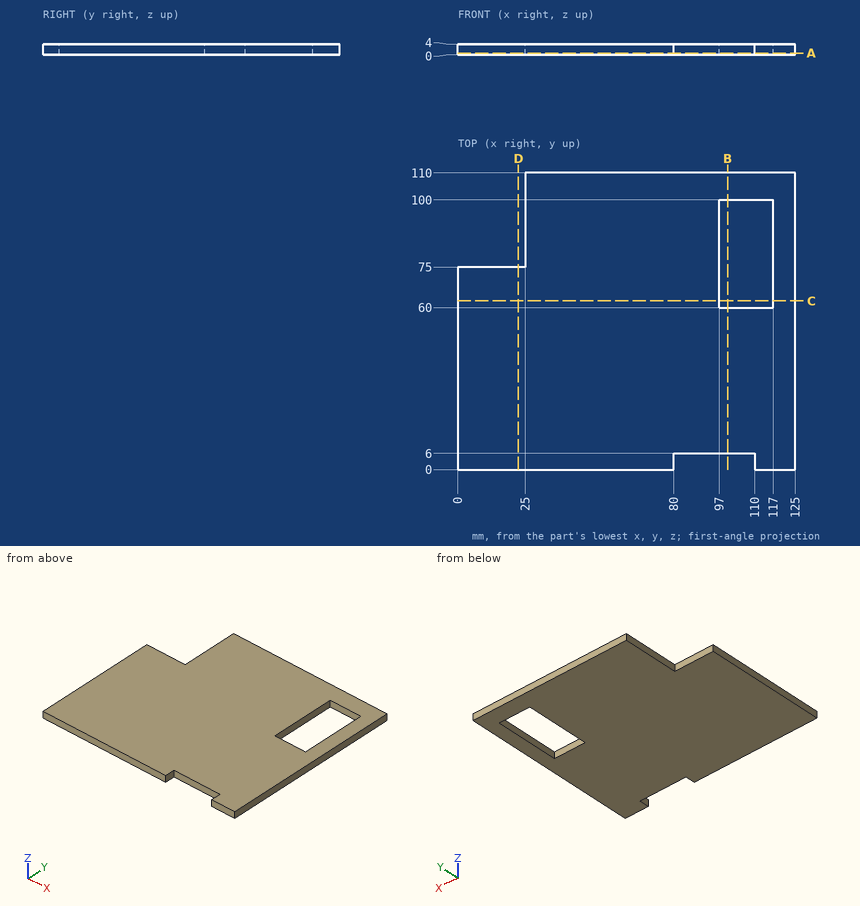
The figure shows three views and two pictorial views of one solid part (mm, origin at its lowest corner). Answer the questions. Coordinates: 2 decimals unless noted, no trailing zeros. Write each loop counter-clockwise with the first axis right and the second up, starting at its lowest first coordinate (ties: lowest second). Pieces come first, ordered by that corner, then holes.
1. The part is cut by section A-A, the plane z = 0.6. Write down the section's boundary in (x, y), and give its area (3 significant figures).
Results list:
outline: (0, 0) - (80, 0) - (80, 6) - (110, 6) - (110, 0) - (125, 0) - (125, 110) - (25, 110) - (25, 75) - (0, 75) - close; hole (97, 60) - (117, 60) - (117, 100) - (97, 100) - close
area: 11,900 mm2
2. The part is cut by section D-D, the plane x = 22.5. Write down the section's boundary in (y, z), and give its area (3 significant figures).
Results list:
outline: (0, 0) - (75, 0) - (75, 4) - (0, 4) - close
area: 300 mm2
3. The part is cut by section C-C, the plane y = 62.5. Write down the section's boundary in (x, z), and give its area (3 significant figures).
Results list:
outline: (0, 0) - (97, 0) - (97, 4) - (0, 4) - close; (117, 0) - (125, 0) - (125, 4) - (117, 4) - close
area: 420 mm2
4. Consider line 1 along X through (y, z) = (85.5, 0.45); line 2 along X through (y, z) = (70.5, 1.3); line 3 along Y through (x, z) = (23, 1.8). Determine where each line is inside the solid, lowest interval first.
Results list:
line 1: x = 25 to 97, 117 to 125
line 2: x = 0 to 97, 117 to 125
line 3: y = 0 to 75
5. Flat-ended cylindrical pins translate along their axes: pin 1 (1 mm diameter, centred on x = 12.5, z = 1, fed in from -Y); pin 2 (1.2 mm diameter, centred on y = 86.5, z = 2, fed in from -X); pin 3 (2 mm diameter, centred on x = 104, z = 1, fed in from -Y); pin 4 (2 mm diameter, centred on x = 17.5, z = 2, fed in from +Y). Find the tip coordinate at first contact, or state that the pin passes through.
Results list:
pin 1: stops at y = 0
pin 2: stops at x = 25
pin 3: stops at y = 6
pin 4: stops at y = 75
6. The part is cut by section B-B, the plane x = 100. Write down the section's boundary in (y, z), and give its area (3 significant figures).
Results list:
outline: (6, 0) - (60, 0) - (60, 4) - (6, 4) - close; (100, 0) - (110, 0) - (110, 4) - (100, 4) - close
area: 256 mm2
